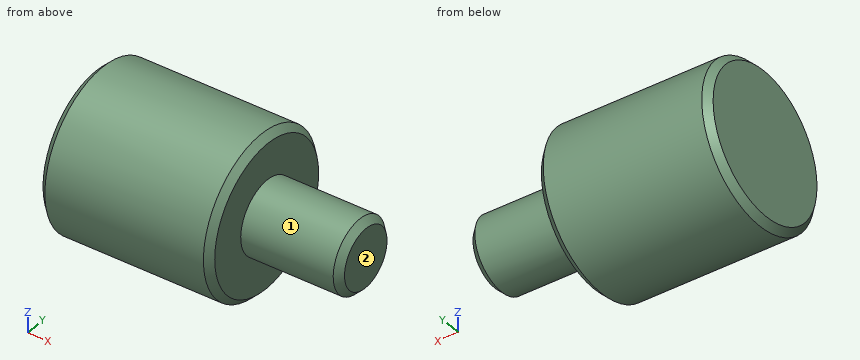
```python
from build123d import *

# Parameters (mm, degrees)
F2_SIZE = 1


with BuildPart() as f1:
    # F0 (on Front) → F1 (revolve)
    with BuildSketch(Plane.XZ):
        Polygon((0, 12), (0, 0), (41, 0), (41, 5.5), (26, 5.5), (26, 12), align=None)
    revolve(axis=Axis((19.196044, 0, 0), (1, 0, 0)))

    # F2
    f2_edges = [f1.edges().sort_by_distance(p)[0] for p in [
        (0, 0, -12),
        (26, 0, -12),
        (41, 0, -5.5),
    ]]
    chamfer(f2_edges, length=F2_SIZE)


solid = f1.part
```
Here's how the part is built. I have some questions about the finished solid (model axes, mm). Face numbers are marked on the shaded views. A direction names the side the tool comes from. Give positions to 0.01 mm unless a question says otherwise; leave off trailing zeros. Write each loop counter-clockwise with the first axis right and the second up, starting at its lowest first coordinate (ties: lowest second). Pieces come first, ordered by that corner, then holes. Notation, with made-up numbers: (-5.75, 41) -> (28.25, 41) arc R15 ccw to (28.25, 64) -> close; hole circle Ø8 at (-3, 47). An arc over 180 degrees is marked (long way). Use one line per item in the form item = value.
1) I'm going to push flat-ended pins straight in: pin 1 (2 mm diameter, centred on y = 8.5, z = 2, fed in from +X); pin 2 (10 mm diameter, centred on x = 25, y = -8, fed in from -Z); pin 3 (3 mm diameter, centred on x = 11.5, z = 8, fed in from -Y). Where does each tip first touch, or does it pass through?
Verdict:
pin_1 = 26
pin_2 = -11.62
pin_3 = -10.09
2) If I drill on L1, parallel to X at y = 8.25, z = -3; L2, parallel to X at y = -5.5, z = -10.5; L3, parallel to Z at x = 6, y = 10.75, over which ranges is the centre line in solid material (lowest first)? Write a range as [from, to].
Verdict:
L1 = [0, 26]
L2 = [0.85, 25.15]
L3 = [-5.33, 5.33]
3) Suppose I cut it at A-A (z = 0). Please give me the cut outline in (x, y), and give its area (3 significant figures).
Verdict:
outline = (0, -11) -> (1, -12) -> (25, -12) -> (26, -11) -> (26, -5.5) -> (40, -5.5) -> (41, -4.5) -> (41, 4.5) -> (40, 5.5) -> (26, 5.5) -> (26, 11) -> (25, 12) -> (1, 12) -> (0, 11) -> close
area = 786 mm2
4) Suppose I cut it at C-C (x = 8.5). Please give me the cut outline in (y, z).
Verdict:
outline = circle Ø24 at (0, 0)
5) Suppose I cut it at D-D (x = 35). Please give me the cut outline in (y, z).
Verdict:
outline = circle Ø11 at (0, 0)
6) On a 3-axis mill with a long thin cutter (end or side, diameter ignored), from which of +Z, -Z, +X, -X, +Y, -Y can I reach the whole of each face in a straight line? I mean the marked faces 1 and 2. Say none if no direction works.
Verdict:
face_1 = +X
face_2 = +Z, -Z, +X, +Y, -Y
